Verification items for the finished model (mm, model axes). Coordinates: 2 decimals unless noted, no trailing zeros. Order: outer loops, then holes, each group sorted by start corner. A loop starts at its lowest first (then second) coordinate and runs counter-clockwise, first axis right, second up. Notation, with made-up numbers: M 87,-32.5 L 99,-32.5 A17 ccw 99,-3.5 Z; hole C -6,-22 d11. An arc over 180 degrees is marked long. Answer as a JSON object with one key per item and string values. Group by question number.
(1) Cross-section at A-A (y = 45). Enter the section's corners in (x, z), plus the area to 3 significant figures.
(2) Material ranges on line 1 (Y direction, x = 20, z = 1.4); line 2 (Y direction, x = -8.5, z = 0.9); line 3 (Y direction, x = 9.5, z = 2.5), recorded low to high.
(3) Cross-section at B-B (y = -6). Enter the section's corners in (x, z).
(4) Gauge pin test, flat ends, axial feed: pin 1 Ø0.9 at (y, z) = (0, 2) entering from -X; pin 2 Ø0.9 at (y, z) = (-7, 2) entering from +X. Record the tip position at first contact, or that the pin passes through.
(5) Cross-section at C-C (x = 3.5). Enter the section's corners in (y, z).
(6) Cross-section at D-D (z = 2). Count the separate pieces of the cut face and the enclosed holes in it, plus the area to 3 significant figures.
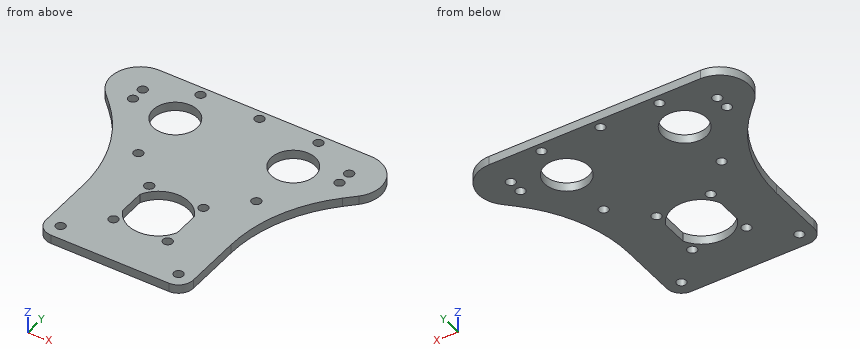
from build123d import *

# Parameters (mm, degrees)
SKETCH_1_W          = 50
SKETCH_1_H          = 50
SKETCH_1_R          = 1.6
EXTRUDE_1_DEPTH     = 3
FILLET_1_R          = 5
CUT_EXTRUDE_1_DEPTH = 36.482389998
EXTRUDE_2_DEPTH     = 3
FILLET_2_R          = 50
SKETCH_4_R          = 1.6
CUT_EXTRUDE_2_DEPTH = 72.672475366
SKETCH_5_R          = 7.5
CUT_EXTRUDE_3_DEPTH = 72.672475366
SKETCH_6_R          = 1.6
CUT_EXTRUDE_4_DEPTH = 72.672475366
SKETCH_7_R          = 1.6
CUT_EXTRUDE_5_DEPTH = 72.672475366


with BuildPart() as part:
    # ｽｹｯﾁ1 → ﾎﾞｽ - 押し出し1 (new body)
    with BuildSketch(Plane.XY):
        Rectangle(SKETCH_1_W, SKETCH_1_H)
        with Locations((-20, 20)):
            Circle(SKETCH_1_R, mode=Mode.SUBTRACT)
        with Locations((-9.192388155, 9.192388155)):
            Circle(SKETCH_1_R, mode=Mode.SUBTRACT)
        with Locations((9.192388155, 9.192388155)):
            Circle(SKETCH_1_R, mode=Mode.SUBTRACT)
        with Locations((20, 20)):
            Circle(SKETCH_1_R, mode=Mode.SUBTRACT)
        with Locations((9.192388155, -9.192388155)):
            Circle(SKETCH_1_R, mode=Mode.SUBTRACT)
        with Locations((20, -20)):
            Circle(SKETCH_1_R, mode=Mode.SUBTRACT)
        with Locations((-9.192388155, -9.192388155)):
            Circle(SKETCH_1_R, mode=Mode.SUBTRACT)
        with Locations((-20, -20)):
            Circle(SKETCH_1_R, mode=Mode.SUBTRACT)
    extrude(amount=EXTRUDE_1_DEPTH)

    # ﾌｨﾚｯﾄ1
    fillet_1_edges = [part.edges().sort_by_distance(p)[0] for p in [
        (25, -25, 1.5),
        (-25, -25, 1.5),
        (-25, 25, 1.5),
        (25, 25, 1.5),
    ]]
    fillet(fillet_1_edges, radius=FILLET_1_R)

    # ｽｹｯﾁ2 → ｶｯﾄ - 押し出し1 (cut, through all)
    with BuildSketch(Plane.XY.offset(3)):
        with BuildLine():
            Line((-9.25, 4.415880433), (-9.25, -4.415880433))
            ThreePointArc((-9.25, -4.415880433), (0, -10.25), (9.25, -4.415880433))
            Line((9.25, -4.415880433), (9.25, 4.415880433))
            ThreePointArc((9.25, 4.415880433), (0, 10.25), (-9.25, 4.415880433))
        make_face()
    extrude(amount=-CUT_EXTRUDE_1_DEPTH, mode=Mode.SUBTRACT)

    # ｽｹｯﾁ3 → ﾎﾞｽ - 押し出し2 (add, through all)
    with BuildSketch(Plane.XY.offset(3)):
        with BuildLine():
            Line((-25, 20), (-42.928932188, 37.928932188))
            ThreePointArc((-42.928932188, 37.928932188), (-45.096659701, 48.826834324), (-35.857864376, 55))
            Line((-35.857864376, 55), (35.857864376, 55))
            ThreePointArc((35.857864376, 55), (45.096659701, 48.826834324), (42.928932188, 37.928932188))
            Line((42.928932188, 37.928932188), (25, 20))
            ThreePointArc((25, 20), (23.535533906, 23.535533906), (20, 25))
            Line((20, 25), (-20, 25))
            ThreePointArc((-20, 25), (-23.535533906, 23.535533906), (-25, 20))
        make_face()
    extrude(amount=-EXTRUDE_2_DEPTH)

    # ﾌｨﾚｯﾄ2
    fillet_2_edges = [part.edges().sort_by_distance(p)[0] for p in [
        (25, 20, 1.5),
        (-25, 20, 1.5),
    ]]
    fillet(fillet_2_edges, radius=FILLET_2_R)

    # ｽｹｯﾁ4 → ｶｯﾄ - 押し出し2 (cut, through all)
    with BuildSketch(Plane.XY.offset(3)):
        with Locations((-35, 45)):
            Circle(SKETCH_4_R)
        with Locations(Location((35, 45, 0), (0, 0, 180))):
            Circle(SKETCH_4_R)
    extrude(amount=-CUT_EXTRUDE_2_DEPTH, mode=Mode.SUBTRACT)

    # ｽｹｯﾁ5 → ｶｯﾄ - 押し出し3 (cut, through all)
    with BuildSketch(Plane.XY.offset(3)):
        with Locations((20, 39)):
            Circle(SKETCH_5_R)
        with Locations(Location((-20, 39, 0), (0, 0, 180))):
            Circle(SKETCH_5_R)
    extrude(amount=-CUT_EXTRUDE_3_DEPTH, mode=Mode.SUBTRACT)

    # ｽｹｯﾁ6 → ｶｯﾄ - 押し出し4 (cut, through all)
    with BuildSketch(Plane(origin=(0, 0, 0), x_dir=(-1, 0, 0), z_dir=(0, 0, -1))):
        with Locations((-35, 40)):
            Circle(SKETCH_6_R)
        with Locations(Location((35, 40, 0), (0, 0, 180))):
            Circle(SKETCH_6_R)
    extrude(amount=-CUT_EXTRUDE_4_DEPTH, mode=Mode.SUBTRACT)

    # ｽｹｯﾁ7 → ｶｯﾄ - 押し出し5 (cut, through all)
    with BuildSketch(Plane.XY.offset(3)):
        with Locations((0, 52)):
            Circle(SKETCH_7_R)
        with Locations((20, 52)):
            Circle(SKETCH_7_R)
        with Locations((-20, 52)):
            Circle(SKETCH_7_R)
    extrude(amount=-CUT_EXTRUDE_5_DEPTH, mode=Mode.SUBTRACT)


solid = part.part
Taken from the geometry:
{
 "1": {"outline": "M -45.86,0 L -36.6,0 L -36.6,3 L -45.86,3 Z; M -33.4,0 L -24.5,0 L -24.5,3 L -33.4,3 Z; M -15.5,0 L 15.5,0 L 15.5,3 L -15.5,3 Z; M 24.5,0 L 33.4,0 L 33.4,3 L 24.5,3 Z; M 36.6,0 L 45.86,0 L 45.86,3 L 36.6,3 Z", "area": "202 mm²"},
 "2": {"line 1": "y = -25 to -21.6, -18.4 to 18.4, 21.6 to 31.5, 46.5 to 50.4, 53.6 to 55", "line 2": "y = -25 to -10.63, -7.75 to -5.73, 5.73 to 7.75, 10.63 to 55", "line 3": "y = -25 to -10.76, -7.62 to 7.62, 10.76 to 55"},
 "3": {"outline": "M -25,0 L -8.31,0 L -8.31,3 L -25,3 Z; M 8.31,0 L 25,0 L 25,3 L 8.31,3 Z"},
 "4": {"pin 1": "stops at x = -25.01", "pin 2": "stops at x = 25"},
 "5": {"outline": "M -25,0 L -9.63,0 L -9.63,3 L -25,3 Z; M 9.63,0 L 55,0 L 55,3 L 9.63,3 Z"},
 "6": {"separate pieces": "1", "enclosed holes": "18", "area": "4,280 mm²"}
}
